Autodesk Inventor part; units mm, degrees
ref_plane "YZ Plane" through (0, 0, 0) normal (1, 0, 0) x (0, 1, 0)
ref_plane "XZ Plane" through (0, 0, 0) normal (0, 1, 0) x (-1, 0, 0)
ref_plane "XY Plane" through (0, 0, 0) normal (0, 0, 1) x (1, 0, 0)
sketch "Sketch1" plane through (0, 0, 0) normal (0, 0, 1) x (1, 0, 0)
  line L0 (-88.5, 34.5) -> (88.5, 34.5)
  line L1 (88.5, 34.5) -> (88.5, -34.5)
  line L2 (88.5, -34.5) -> (-88.5, -34.5)
  line L3 (-88.5, -34.5) -> (-88.5, 34.5)
  point P0 (0, 0)
  point P1 (-88.5, 0)
  point P2 (0, 34.5)
  dimension "d0" = 177
  dimension "d1" = 69
sketch "Sketch1 outline for Extrusion1" plane through (0, 0, 0) normal (0, 0, 1) x (1, 0, 0)
  line L0 (-88.5, -34.5) -> (88.5, -34.5)
  line L1 (-88.5, 34.5) -> (-88.5, -34.5)
  line L2 (88.5, 34.5) -> (-88.5, 34.5)
  line L3 (88.5, -34.5) -> (88.5, 34.5)
extrude "Extrusion1" add sketch "Sketch1 outline for Extrusion1" along normal blind 65
sketch "Sketch2" plane through (0, 0, 0) normal (0, 0, -1) x (-1, 0, 0)
  line L0 (232.5, 3.5) -> (-12.5, 3.5)
  line L1 (88.5, 34.5) -> (88.5, -34.5)
  line L2 (-88.5, 34.5) -> (88.5, 34.5)
  line L3 (-22.5, 34.5) -> (-22.5, 3.5)
  line L4 (-22.5, 13.5) -> (-22.5, 24.5)
  line L5 (-12.5, 3.5) -> (-22.5, 3.5)
  point P0 (0, 0)
  point P1 (88.5, 3.5)
sketch "Sketch2 outline for Extrusion2" plane through (0, 0, 0) normal (0, 0, -1) x (-1, 0, 0)
  line L0 (-22.5, 3.5) -> (-12.5, 3.5)
  line L1 (-22.5, 34.5) -> (-22.5, 3.5)
  line L2 (88.5, 34.5) -> (-22.5, 34.5)
  line L3 (88.5, 3.5) -> (88.5, 34.5)
  line L4 (-12.5, 3.5) -> (88.5, 3.5)
extrude "Extrusion2" cut sketch "Sketch2 outline for Extrusion2" against normal through all
fillet "Fillet1" radius 10 2 edges at (22.5, 3.5, 32.5) (22.5, 34.5, 32.5)
sketch "Sketch3" plane through (0, 0, 0) normal (0, 0, -1) x (-1, 0, 0)
  line L0 (-43.5, -11.5) -> (216.5, -11.5)
  line L1 (-43.5, 32.5) -> (-43.5, -11.5)
  line L2 (-90.5, 32.5) -> (-43.5, 32.5)
  line L3 (-88.5, 32.5) -> (-88.5, -34.5)
  line L4 (-88.5, -34.5) -> (88.5, -34.5)
  line L5 (88.5, -34.5) -> (88.5, -11.5)
  line L6 (88.5, 3.5) -> (88.5, -34.5)
  line L7 (88.5, -34.5) -> (-88.5, -34.5)
  line L8 (-88.5, -34.5) -> (-88.5, 34.5)
  point P0 (0, 0)
sketch "Sketch3 outline for Extrusion3" plane through (0, 0, 0) normal (0, 0, -1) x (-1, 0, 0)
  line L0 (-43.5, -11.5) -> (-43.5, 32.5)
  line L1 (88.5, -11.5) -> (-43.5, -11.5)
  line L2 (88.5, -34.5) -> (88.5, -11.5)
  line L3 (-88.5, -34.5) -> (88.5, -34.5)
  line L4 (-88.5, 32.5) -> (-88.5, -34.5)
  line L5 (-43.5, 32.5) -> (-88.5, 32.5)
extrude "Extrusion3" cut sketch "Sketch3 outline for Extrusion3" against normal blind 60
sketch "Sketch4" plane through (88.5, 34.5, 65) normal (0, 1, 0) x (1, 0, 0)
  line L0 (0, 65) -> (-56, 65)
  line L1 (0, 65) -> (0, 0)
  line L2 (0, 40) -> (-25, 65)
  line L3 (0, 38.585786) -> (-26.414214, 65)
  point P0 (-88.5, 65)
  dimension "d40" = 1
sketch "Sketch4 outline for Extrusion4" plane through (88.5, 34.5, 65) normal (0, 1, 0) x (1, 0, 0)
  line L0 (0, 65) -> (-26.414214, 65)
  line L1 (-26.414214, 65) -> (0, 38.585786)
  line L2 (0, 38.585786) -> (0, 65)
extrude "Extrusion4" cut sketch "Sketch4 outline for Extrusion4" against normal blind 60
sketch "Sketch5" plane through (0, 0, 65) normal (0, 0, 1) x (1, 0, 0)
  line L0 (50.5, -5.5) -> (55.5, -5.5)
  line L1 (55.5, -5.5) -> (55.5, 9.5)
  line L2 (55.5, 9.5) -> (50.5, 9.5)
  line L3 (50.5, 9.5) -> (50.5, -5.5)
  line L4 (-88.5, -34.5) -> (88.5, -34.5)
  line L5 (88.5, -34.5) -> (88.5, 34.5)
  line L6 (55.5, 9.5) -> (60.5, 9.5)
  line L7 (60.5, 9.5) -> (60.5, 4.5)
  line L8 (60.5, 4.5) -> (55.5, 4.5)
  line L9 (55.5, 4.5) -> (55.5, 9.5)
  line L10 (55.5, 19.5) -> (60.5, 19.5)
  line L11 (60.5, 19.5) -> (60.5, 9.5)
  line L12 (60.5, 9.5) -> (55.5, 9.5)
  line L13 (55.5, 9.5) -> (55.5, 19.5)
  line L14 (50.5, 19.5) -> (55.5, 19.5)
  line L15 (55.5, 19.5) -> (55.5, 14.5)
  line L16 (55.5, 14.5) -> (50.5, 14.5)
  line L17 (50.5, 14.5) -> (50.5, 19.5)
  line L18 (50.5, 34.5) -> (55.5, 34.5)
  line L19 (55.5, 34.5) -> (55.5, 19.5)
  line L20 (55.5, 19.5) -> (50.5, 19.5)
  line L21 (50.5, 19.5) -> (50.5, 34.5)
  line L22 (88.5, 34.5) -> (32.5, 34.5)
  point P0 (0, 0)
  dimension "d11" = 5
  dimension "d13" = 33
  dimension "d20" = 5
  dimension "d21" = 10
  dimension "d23" = 15
  dimension "d24" = 15
sketch "Sketch5 outline for Extrusion5" plane through (0, 0, 65) normal (0, 0, 1) x (1, 0, 0)
  line L0 (55.5, 9.5) -> (50.5, 9.5)
  line L1 (50.5, 9.5) -> (50.5, -5.5)
  line L2 (50.5, -5.5) -> (55.5, -5.5)
  line L3 (55.5, -5.5) -> (55.5, 4.5)
  line L4 (55.5, 4.5) -> (60.5, 4.5)
  line L5 (60.5, 4.5) -> (60.5, 19.5)
  line L6 (60.5, 19.5) -> (55.5, 19.5)
  line L7 (55.5, 19.5) -> (55.5, 34.5)
  line L8 (55.5, 34.5) -> (50.5, 34.5)
  line L9 (50.5, 34.5) -> (50.5, 14.5)
  line L10 (50.5, 14.5) -> (55.5, 14.5)
  line L11 (55.5, 14.5) -> (55.5, 9.5)
extrude "Extrusion5" cut sketch "Sketch5 outline for Extrusion5" against normal blind 30
sketch "Sketch6" plane through (0, 0, 0) normal (0, 0, -1) x (-1, 0, 0)
  line L0 (-28.5, 18.5) -> (-33.5, 18.5)
  line L1 (-33.5, 18.5) -> (-33.5, 8.5)
  line L2 (-28.5, 8.5) -> (-28.5, 18.5)
  line L3 (-33.5, 8.5) -> (-28.5, 8.5)
  line L4 (54.5, -1.5) -> (4.5, -1.5)
  line L5 (4.5, -1.5) -> (4.5, -6.5)
  line L6 (4.5, -6.5) -> (54.5, -6.5)
  line L7 (54.5, -6.5) -> (54.5, -1.5)
  line L8 (4.65, -1.65) -> (54.35, -1.65)
  line L9 (54.35, -1.65) -> (54.35, -6.35)
  line L10 (54.35, -6.35) -> (4.65, -6.35)
  line L11 (4.65, -6.35) -> (4.65, -1.65)
  line L12 (-33.35, 8.65) -> (-33.35, 18.35)
  line L13 (-33.35, 18.35) -> (-28.65, 18.35)
  line L14 (-28.65, 18.35) -> (-28.65, 8.65)
  line L15 (-28.65, 8.65) -> (-33.35, 8.65)
  line L16 (-33.35, 16.85) -> (-28.65, 16.85)
  line L17 (-33.35, 10.15) -> (-28.65, 10.15)
  line L18 (6.65, -6.35) -> (6.65, -1.65)
  line L19 (52.35, -6.35) -> (52.35, -1.65)
  point P0 (0, 0)
  dimension "d17" = 0.15
  dimension "d35" = 0.15
  dimension "d36" = 1.5
  dimension "d37" = 1.5
  dimension "d38" = 2
  dimension "d39" = 2
sketch "Sketch6 outline for Extrusion6" plane through (0, 0, 0) normal (0, 0, -1) x (-1, 0, 0)
  line L0 (-33.35, 10.15) -> (-28.65, 10.15)
  line L1 (-33.35, 16.85) -> (-33.35, 10.15)
  line L2 (-28.65, 16.85) -> (-33.35, 16.85)
  line L3 (-28.65, 10.15) -> (-28.65, 16.85)
  line L4 (52.35, -6.35) -> (52.35, -1.65)
  line L5 (6.65, -6.35) -> (52.35, -6.35)
  line L6 (6.65, -1.65) -> (6.65, -6.35)
  line L7 (52.35, -1.65) -> (6.65, -1.65)
extrude "Extrusion6" add sketch "Sketch6 outline for Extrusion6" along normal blind 8
fillet "Fillet2" radius 10 6 edges at (72, 34.5, 65) (25.4289, 31.5711, 65) (22.5, 19, 65) (19.5711, 6.4289, 65) (-38, 3.5, 65) (41.5, 34.5, 65)
sketch "Sketch7" plane through (32.5, 34.5, 0) normal (0, 1, 0) x (1, 0, 0)
  line L0 (32, -48) -> (12, -48)
  line L1 (12, -48) -> (12, -35)
  line L2 (12, -35) -> (32, -35)
  line L3 (32, -35) -> (32, -48)
  line L4 (18, -35) -> (23, -35)
  point P0 (-32.5, 0)
  point P1 (20.5, -35)
  dimension "d26" = 20
  dimension "d27" = 13
sketch "Sketch7 outline for Extrusion7" plane through (32.5, 34.5, 0) normal (0, 1, 0) x (1, 0, 0)
  line L0 (12, -35) -> (12, -48)
  line L1 (32, -35) -> (12, -35)
  line L2 (32, -48) -> (32, -35)
  line L3 (12, -48) -> (32, -48)
extrude "Extrusion7" cut sketch "Sketch7 outline for Extrusion7" against normal blind 30
move faces "Move1" translate (-1, 0, 0) faces at (88.5, 7.5, 61.666667)
fillet "Fillet3" radius 10 2 edges at (71.5, 32.5, 60) (47, 32.5, 60)
properties part number "0008-30-011"
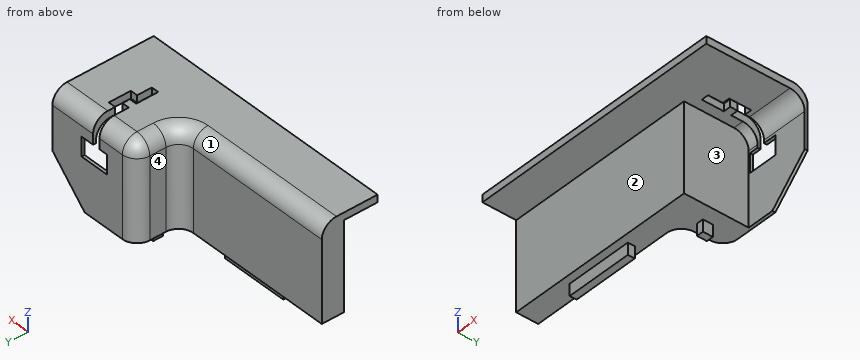
Here's how the part is built. I have some questions about the finished solid (model axes, mm). Face numbers are marked on the shaded views. A direction names the side the tool comes from. Coordinates: 2 decimals unless noted, no trailing zeros. Loops run counter-clockwise (first coordinate to the right, second up) from the corner with the lowest first, then second, coordinate; pieces in that order, holes last.
1. Imagine slicing it at B-B, the plane x = 53.5. Please give me the cut outline in (y, z).
2. For the marked faces 1, 2, 3 and 4, which set-ups out of +Z, -Z, +X, -X, +Y, -Y let a thin tool reach every point of the face, with its end or its side?
3. Imagine slicing it at D-D, the plane y = 29. Please give me the cut outline in (x, z), and give its area (3 significant figures).
4. For P1, Ø1.6, axis at x = 58.5, y = 33.5, coming from the -Z side; P2, Ø5, axis at x = -56, z = 52, coming from the +Y side; P3, Ø2.5, axis at x = -28.5, z = -6, coming from the -Y side, each with a flat end and sliding along its axis, tell me the tip position at first contact or that it passes through.
5. Imagine slicing it at C-C, the plane x = -49. Please give me the cut outline in (y, z).
6. I need wall thicknesses on L1, parallel to X at y = -10, z = 15; L2, parallel to Y at x = 34, z = 50; L3, parallel to Z at x = 75, y = 22. Which ranges of each line are inside material? Lowest first, please.
7. Imagine slicing it at A-A, the plane z = 40.5. Please give me the cut outline in (x, y).
Taken from the geometry:
1. outline: (-34.5, 60) - (-5.5, 60) - (-5.5, 65) - (-34.5, 65) - close; (9.5, 60) - (14.5, 60) - (14.5, 65) - (9.5, 65) - close; (32.5, 0) - (34.5, 0) - (34.5, 35) - (32.5, 35) - close
2. face 1: +Z, -X, +Y
2. face 2: -Z, +X, -X, -Y
2. face 3: -Z, +X, -Y
2. face 4: +Z, -Z, -X, +Y
3. outline: (23.57, 0) - (43.5, 0) - (43.5, 57.6) - (50.5, 57.6) - (50.5, 63.93) - (32.5, 63.93) arc R8.93 ccw to (23.57, 55) - close; (55.5, 57.6) - (87.5, 57.6) - (87.5, 63.93) - (55.5, 63.93) - close
3. area: 1,500 mm2
4. P1: stops at z = 0
4. P2: stops at y = 3.5
4. P3: stops at y = -6.35
5. outline: (-34.5, 60) - (-11.5, 60) - (-11.5, 0) - (-6.35, 0) - (-6.35, -8) - (-1.65, -8) - (-1.65, 0) - (3.5, 0) - (3.5, 55) arc R10 ccw to (-6.5, 65) - (-34.5, 65) - close
6. L1: x = -88.5 to 43.5
6. L2: y = -11.5 to 34.5
6. L3: z = 60 to 65
7. outline: (-88.5, -11.5) - (43.5, -11.5) - (43.5, 32.5) - (44.5, 32.5) - (44.5, 34.5) - (32.5, 34.5) arc R10 ccw to (22.5, 24.5) - (22.5, 13.5) arc R10 cw to (12.5, 3.5) - (-88.5, 3.5) - close; (64.5, 32.5) - (87.5, 32.5) - (87.5, 34.5) - (64.5, 34.5) - close
